Geometry check sheet. Reference: the model listing, model coordinates, mm. A direction names the side the tool comes from. Round coordinates to 2 decimals unless told otherwise and drop trailing zeros. Write each loop counter-clockwise with the first axis right and the second up, starting at its lowest first coordinate (ties: lowest second). Pieces come first, ordered by that corner, then holes.
Item 1: Cross-section at B-B (z = 46.5). Enter the section's corners in (x, y), then the cut area to 3 significant figures.
Item 2: Access from +Z, -Z, +X, -X, +Y, -Y to the whole of each face (thin tool, end or side, straight path). Record for faces 1 (the face through (-1, -545.338, -35)), 2 (the face through (31, -9.827, 31)), 3 (the face through (-6.883, -366.646, -30.995)).
Item 3: Depth check by flat-ended pin: P1, Ø12, axis at x = -31, y = -345, coming from the +Z side; P2, Ø3, axis at x = 47.5, y = -5.5, coming from the +Z side; P3, Ø6, axis at y = -396.5, z = 16, coming from the -X side. Enter the tip coordinate at first touch or a pass-through.
Item 4: Cross-section at A-A (y = -250). Enter the section's corners in (x, z).
Item 5: Cross-section at C-C (y = -76.5). Enter the section's corners in (x, z).
Item 6: Scan lines: probe 1 along Z at (x, y) = (1, -514); probe 2 along Y at (x, z) = (16.5, 34.5); probe 3 along Z at (x, y) = (-9, -484). Record each from-to range of solid material in increasing order.
Item 7: Cross-section at D-D (x = 71.5). Enter the section's corners in (y, z), then the cut area to 3 significant figures.
Item 8: Draft check along Z on faces 4 (the face through (-19, 0, -17)), 5 (the face through (0, -175.26, 0)), 6 (the face through (-10.675, -268.852, 81.306)). Enter one of: pulls with the +Z half, pulls with the -Z half, needs draft (parallel to the pull), parting line crosses it, or undercut.
from build123d import *

# Parameters (mm, degrees)
F0_R     = 82.0039
F1_DEPTH = 545.338
F2_R     = 31.75
F3_DEPTH = 370.078
F4_R     = 7.62
F5_W     = 9.82706
F5_H     = 91.064006
F6_DEPTH = 117


with BuildPart() as f1:
    # F0 (on Front) → F1 (new body)
    with BuildSketch(Plane.XZ):
        Circle(F0_R)
    extrude(amount=F1_DEPTH)

    # F2 (on face) → F3 (cut)
    with BuildSketch(Plane.XZ.offset(545.338)):
        Circle(F2_R)
    extrude(amount=-F3_DEPTH, mode=Mode.SUBTRACT)

    # F4
    f4_edges = [f1.edges().sort_by_distance(p)[0] for p in [
        (-31.75, -175.26, 0),
    ]]
    fillet(f4_edges, radius=F4_R)

    # F5 (on Right) → F6 (cut)
    with BuildSketch(Plane.YZ):
        with Locations((-4.91353, 45.532003)):
            Rectangle(F5_W, F5_H)
    extrude(amount=F6_DEPTH, mode=Mode.SUBTRACT)


solid = f1.part
Resolved:
1. outline: (-67.55, -545.34) - (67.55, -545.34) - (67.55, -9.83) - (0, -9.83) - (0, 0) - (-67.55, 0) - close
1. area: 73,000 mm2
2. face 1: +Z, -Z, +X, -X, -Y
2. face 2: +Z, +X, +Y
2. face 3: -Y
3. P1: stops at z = 78.1
3. P2: stops at z = 0
3. P3: stops at x = -80.97
4. outline: circle Ø164.01 at (0, 0); hole circle Ø63.5 at (0, 0)
5. outline: circle Ø164.01 at (0, 0)
6. probe 1: z = -82 to -31.73, 31.73 to 82
6. probe 2: y = -545.34 to -9.83
6. probe 3: z = -81.51 to -30.45, 30.45 to 81.51
7. outline: (-545.34, -40.15) - (0, -40.15) - (0, 0) - (-9.83, 0) - (-9.83, 40.15) - (-545.34, 40.15) - close
7. area: 43,400 mm2
8. face 4: needs draft
8. face 5: undercut
8. face 6: parting line crosses it
